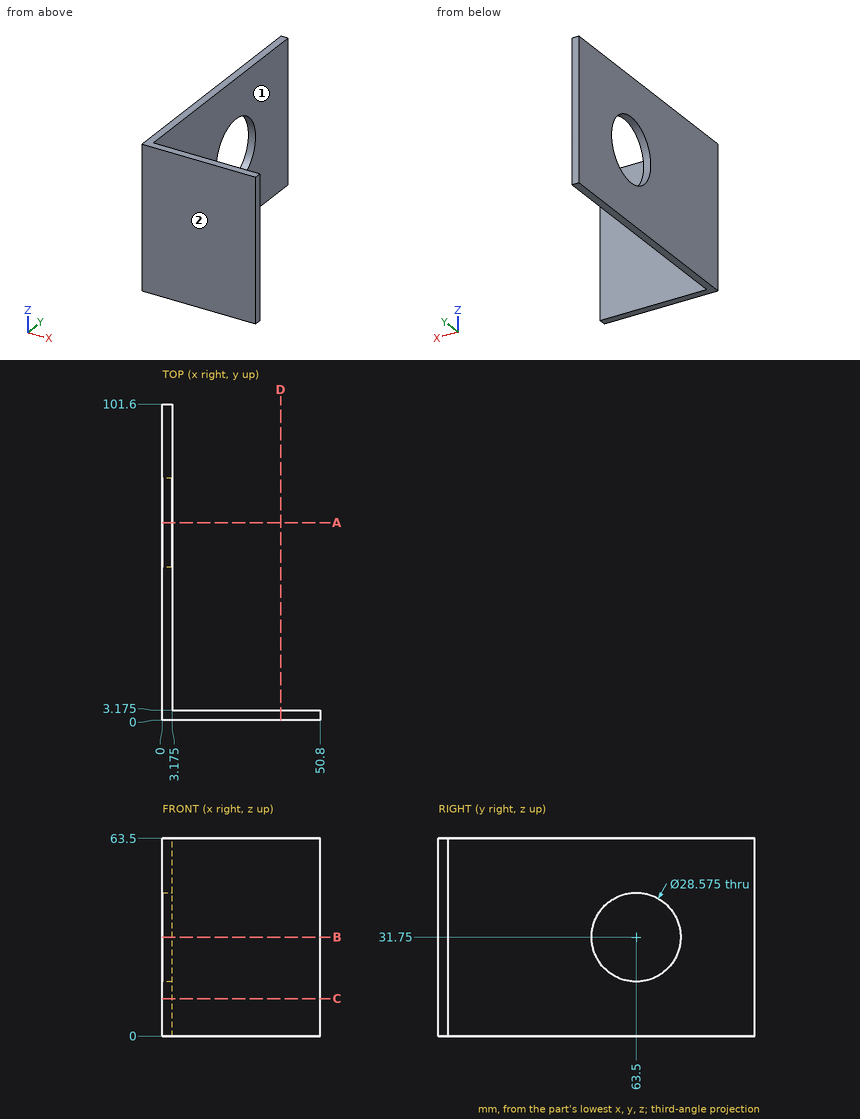
For this review, use the dimensioned drawing (mm, ordinates from the lowest corner) and the shaded views. A direction names the side the tool comes from. Give positions to 0.01 mm unless a question says otherwise; leave off trailing zeros. Write each loop counter-clockwise with the first axis right and the second up, starting at its lowest first coordinate (ties: lowest second). Pieces come first, ordered by that corner, then holes. Notation, with made-up numbers: M 43.5,20 L 57.5,20 A35 ccw 57.5,58 Z; hole C 2.5,67.5 d11. An arc over 180 degrees is marked long. Answer as a JSON object with one key per item and string values. Group by question number.
Item 1: Consider section D-D on x = 38. Write out the cut boundary in (y, z) (3 decimals).
Item 2: Consider section C-C on z = 12. Write out the cut boundary in (x, y) (3 decimals), plus the area to 3 significant figures.
Item 3: Tool access review of the marked faces 1 and 2: name each direction out of +Z, -Z, +X, -X, +Y, -Y from which nothing blocks a thin tool from reaching the whole face with its end or side.
Item 4: Consider section B-B on z = 31.75. Write out the cut boundary in (x, y) (1 decimal).
Item 5: Consider section A-A on y = 63.5. Write out the cut boundary in (x, z) (1 decimal).
Item 6: For pin 1 Ø3 at (x, z) = (29.5, 21.5) entering from +Y (3 decimals); pin 2 Ø4 at (y, z) = (90.5, 37) entering from +X (3 decimals), all flat-tipped, find the tip position at first contact; note any pin that passes through.
Item 7: For probe 1 along Z at (x, y) = (1, 63); probe 2 along Y at (x, z) = (24, 15) (3 decimals), list the stretches that pass through material, from the lowest coordinate up. Write a range as [from, to].
Check result:
{
 "1": {"outline": "M 0,0 L 3.175,0 L 3.175,63.5 L 0,63.5 Z"},
 "2": {"outline": "M 0,0 L 50.8,0 L 50.8,3.175 L 3.175,3.175 L 3.175,101.6 L 0,101.6 Z", "area": "474 mm^2"},
 "3": {"face 1": "+Z, -Z, +X, +Y", "face 2": "+Z, -Z, +X, -X, -Y"},
 "4": {"outline": "M 0,0 L 50.8,0 L 50.8,3.2 L 3.2,3.2 L 3.2,49.2 L 0,49.2 Z; M 0,77.8 L 3.2,77.8 L 3.2,101.6 L 0,101.6 Z"},
 "5": {"outline": "M 0,0 L 3.2,0 L 3.2,17.5 L 0,17.5 Z; M 0,46 L 3.2,46 L 3.2,63.5 L 0,63.5 Z"},
 "6": {"pin 1": "stops at y = 3.175", "pin 2": "stops at x = 3.175"},
 "7": {"probe 1": "z = [0, 17.47], [46.03, 63.5]", "probe 2": "y = [0, 3.175]"}
}
